from build123d import *

# Parameters (mm, degrees)
F1_DEPTH = 25.4


with BuildPart() as f1:
    # F0 (on Front) → F1 (new body, symmetric)
    with BuildSketch(Plane.XZ):
        with BuildLine():
            Line((-88.9, 0), (0, 0))
            Line((0, 0), (88.9, 0))
            Line((88.9, 0), (88.9, 53.086))
            Line((88.9, 53.086), (86.868, 53.086))
            ThreePointArc((86.868, 53.086), (84.533133, 52.118867), (83.566, 49.784))
            Line((83.566, 49.784), (83.566, 13.208))
            ThreePointArc((83.566, 13.208), (81.259759, 7.640241), (75.692, 5.334))
            Line((75.692, 5.334), (-75.692, 5.334))
            ThreePointArc((-75.692, 5.334), (-81.259759, 7.640241), (-83.566, 13.208))
            Line((-83.566, 13.208), (-83.566, 49.784))
            ThreePointArc((-83.566, 49.784), (-84.533133, 52.118867), (-86.868, 53.086))
            Line((-86.868, 53.086), (-88.9, 53.086))
            Line((-88.9, 53.086), (-88.9, 0))
        make_face()
    extrude(amount=F1_DEPTH, both=True)


solid = f1.part
Model file for the job. Use its own axes, mm. A direction names the side the tool comes from. Give positions to 0.01 mm unless a question says otherwise; leave off trailing zeros. Loops run counter-clockwise (first coordinate to the right, second up) from the corner with the lowest first, then second, coordinate; pieces in that order, holes last.
1) Wall check: line 1 (X direction, y = 3, z = 31.5); line 2 (Z direction, x = -31.5, y = 3); line 3 (X direction, y = -19.5, z = 10). Give the ranges that are in metal, low to high.
2) Tool access for faces 1 (the flat face through (83.566, 0, 32)), 2 (the flat face through (88.9, 0, 26)): list every direction of +Z, -Z, +X, -X, +Y, -Y with a clear straight run to the whole face (end or side of a thin tool).
3) Saw through at B-B (y = -7). Write the cut outline in (x, z), plus the area to 3 significant figures.
4) Flat gauge pin, fed straight in: pin 1 Ø1 at (x, y) = (45, -17) entering from +Z. Where does the tip first touch, or does it go through?
5) Saw through at D-D (z = 11). Write the cut outline in (x, y).
6) Saw through at C-C (x = 67.5). Write the cut outline in (y, z), plus the area to 3 significant figures.
7) Saw through at A-A (z = 26). Write the cut outline in (x, y).
8) Pull direction X, two halves, no side cores. Call faces 3 (the flat face through (-83.566, 0, 31)), 4 (the flat face through (0, 25.4, 3)), 5 (the flat face through (-88.9, 0, 27)): +X half, -X half, draft (parallel to the pull), parting line (faces both ways), or undercut.
Answer block:
1. line 1: x = -88.9 to -83.57, 83.57 to 88.9
1. line 2: z = 0 to 5.33
1. line 3: x = -88.9 to -82.88, 82.88 to 88.9
2. face 1: +Z, +Y, -Y
2. face 2: +Z, -Z, +X, +Y, -Y
3. outline: (-88.9, 0) - (88.9, 0) - (88.9, 53.09) - (86.87, 53.09) arc R3.3 ccw to (83.57, 49.78) - (83.57, 13.21) arc R7.87 cw to (75.69, 5.33) - (-75.69, 5.33) arc R7.87 cw to (-83.57, 13.21) - (-83.57, 49.78) arc R3.3 ccw to (-86.87, 53.09) - (-88.9, 53.09) - close
3. area: 1,480 mm2
4. pin 1: stops at z = 5.33
5. outline: (-88.9, -25.4) - (-83.25, -25.4) - (-83.25, 25.4) - (-88.9, 25.4) - close; (83.25, -25.4) - (88.9, -25.4) - (88.9, 25.4) - (83.25, 25.4) - close
6. outline: (-25.4, 0) - (25.4, 0) - (25.4, 5.33) - (-25.4, 5.33) - close
6. area: 271 mm2
7. outline: (-88.9, -25.4) - (-83.57, -25.4) - (-83.57, 25.4) - (-88.9, 25.4) - close; (83.57, -25.4) - (88.9, -25.4) - (88.9, 25.4) - (83.57, 25.4) - close
8. face 3: undercut
8. face 4: draft
8. face 5: -X half
